from build123d import *

# Parameters (mm, degrees)
F1_DEPTH  = 2
F2_R      = 1.5
F3_DEPTH  = 5
F4_R      = 19
F5_DEPTH  = 27
F6_W      = 47
F6_H      = 27
F7_DEPTH  = 5
F8_W      = 47
F8_H      = 5
F9_DEPTH  = 120
F11_DEPTH = 10
F13_DEPTH = 25
F15_DEPTH = 25
F16_R     = 5


with BuildPart() as f1:
    # F0 (on Front) → F1 (new body)
    with BuildSketch(Plane.XZ):
        with BuildLine():
            Line((-23.5, -23.5), (0, -23.5))
            Line((0, -23.5), (23.5, -23.5))
            Line((23.5, -23.5), (23.5, 0))
            ThreePointArc((23.5, 0), (0, 23.5), (-23.5, 0))
            Line((-23.5, 0), (-23.5, -23.5))
        make_face()
    extrude(amount=F1_DEPTH)

    # F2 (on face) → F3 (cut)
    with BuildSketch(Plane.XZ.offset(2)):
        with Locations((15.5, 0)):
            Circle(F2_R)
        with Locations((7.75, 13.423394)):
            Circle(F2_R)
        with Locations((-7.75, 13.423394)):
            Circle(F2_R)
        with Locations((-15.5, 0)):
            Circle(F2_R)
        with Locations((-7.75, -13.423394)):
            Circle(F2_R)
        with Locations((7.75, -13.423394)):
            Circle(F2_R)
        with BuildLine():
            Line((6.5, -7), (6.5, 7))
            ThreePointArc((6.5, 7), (0, 13.5), (-6.5, 7))
            Line((-6.5, 7), (-6.5, -7))
            ThreePointArc((-6.5, -7), (0, -13.5), (6.5, -7))
        make_face()
    extrude(amount=-F3_DEPTH, mode=Mode.SUBTRACT)

    # F4 (on Front) → F5 (join)
    with BuildSketch(Plane.XZ):
        with BuildLine():
            ThreePointArc((23.5, 0), (0, 23.5), (-23.5, 0))
            Line((-23.5, 0), (-23.5, -23.5))
            Line((-23.5, -23.5), (23.5, -23.5))
            Line((23.5, -23.5), (23.5, 0))
        make_face()
        with Locations((0, -0.678439)):
            Circle(F4_R, mode=Mode.SUBTRACT)
    extrude(amount=F5_DEPTH)

    # F6 (on face) → F7 (join)
    with BuildSketch(Plane(origin=(0, 0, -23.5), x_dir=(1, 0, 0), z_dir=(0, 0, -1))):
        with Locations((0, 13.5)):
            Rectangle(F6_W, F6_H)
    extrude(amount=F7_DEPTH)

    # F8 (on face) → F9 (join)
    with BuildSketch(Plane(origin=(0, 0, -28.5), x_dir=(1, 0, 0), z_dir=(0, 0, -1))):
        with Locations((0, 2.5)):
            Rectangle(F8_W, F8_H)
    extrude(amount=F9_DEPTH)

    # F10 (on face) → F11 (join)
    with BuildSketch(Plane.XZ.offset(5)):
        Polygon((-2.6, -51), (-2.6, -43.5), (-2.6, -36), (-7.6, -36), (-7.6, -51), align=None)
        Polygon((2.6, -126), (2.6, -133.5), (2.6, -141), (7.6, -141), (7.6, -126), align=None)
        Polygon((2.6, -36), (2.6, -43.5), (2.6, -51), (7.6, -51), (7.6, -36), align=None)
        Polygon((-2.6, -141), (-2.6, -133.5), (-2.6, -126), (-7.6, -126), (-7.6, -141), align=None)
    extrude(amount=F11_DEPTH)

    # F12 (on face) → F13 (cut)
    with BuildSketch(Plane.YZ.offset(7.6)):
        with BuildLine():
            ThreePointArc((-9.16795, -42.251925), (-10, -42), (-10.83205, -42.251925))
            Line((-10.83205, -42.251925), (-10, -43.5))
            Line((-10, -43.5), (-9.16795, -42.251925))
        make_face()
        with BuildLine():
            Line((-10, -43.5), (-10.83205, -42.251925))
            ThreePointArc((-10.83205, -42.251925), (-11.5, -43.5), (-10.83205, -44.748075))
            Line((-10.83205, -44.748075), (-10, -43.5))
        make_face()
        with BuildLine():
            Line((-9.16795, -42.251925), (-10, -43.5))
            Line((-10, -43.5), (-9.16795, -44.748075))
            ThreePointArc((-9.16795, -44.748075), (-8.677488, -44.207787), (-8.5, -43.5))
            ThreePointArc((-8.5, -43.5), (-8.677488, -42.792213), (-9.16795, -42.251925))
        make_face()
        with BuildLine():
            Line((-9.16795, -44.748075), (-10, -43.5))
            Line((-10, -43.5), (-10.83205, -44.748075))
            ThreePointArc((-10.83205, -44.748075), (-10, -45), (-9.16795, -44.748075))
        make_face()
    extrude(amount=-F13_DEPTH, mode=Mode.SUBTRACT)

    # F14 (on face) → F15 (cut)
    with BuildSketch(Plane.YZ.offset(7.6)):
        with BuildLine():
            ThreePointArc((-9.16795, -132.251925), (-10, -132), (-10.83205, -132.251925))
            Line((-10.83205, -132.251925), (-10, -133.5))
            Line((-10, -133.5), (-9.16795, -132.251925))
        make_face()
        with BuildLine():
            Line((-10, -133.5), (-10.83205, -132.251925))
            ThreePointArc((-10.83205, -132.251925), (-11.5, -133.5), (-10.83205, -134.748075))
            Line((-10.83205, -134.748075), (-10, -133.5))
        make_face()
        with BuildLine():
            Line((-9.16795, -132.251925), (-10, -133.5))
            Line((-10, -133.5), (-9.16795, -134.748075))
            ThreePointArc((-9.16795, -134.748075), (-8.677488, -134.207787), (-8.5, -133.5))
            ThreePointArc((-8.5, -133.5), (-8.677488, -132.792213), (-9.16795, -132.251925))
        make_face()
        with BuildLine():
            Line((-9.16795, -134.748075), (-10, -133.5))
            Line((-10, -133.5), (-10.83205, -134.748075))
            ThreePointArc((-10.83205, -134.748075), (-10, -135), (-9.16795, -134.748075))
        make_face()
    extrude(amount=-F15_DEPTH, mode=Mode.SUBTRACT)

    # F16
    f16_edges = [f1.edges().sort_by_distance(p)[0] for p in [
        (5.1, -15, -141),
        (5.1, -15, -126),
        (-5.1, -15, -126),
        (-5.1, -15, -141),
        (5.1, -15, -51),
        (5.1, -15, -36),
        (-5.1, -15, -36),
        (-5.1, -15, -51),
    ]]
    fillet(f16_edges, radius=F16_R)


solid = f1.part
Work out the finished part from the listing and answer in its coordinate system (mm). A direction names the side the tool comes from. Give positions to 0.01 mm unless a question says otherwise; leave off trailing zeros. Order: outer loops, then holes, each group sorted by start corner. A loop starts at its lowest first (then second) coordinate and runs counter-clockwise, first axis right, second up. Notation, with made-up numbers: (-19, -6.5) -> (32, -6.5) arc R28 cw to (32, 23.5) -> close; hole circle Ø1 at (23.5, 29.5). An arc over 180 degrees is marked (long way). Answer as a JSON object with one key per item and string values. Group by question number.
1. Section A-A on x = 0 is taken. Determine the outline of the cut face in (y, z).
2. Section C-C on z = -53.5 is taken. Determine the outline of the cut face in (x, y), plus the area to 3 significant figures.
3. Section B-B on y = -25.5 is taken. Determine the outline of the cut face in (x, z), plus the area to 3 significant figures.
4. The mould has two halves that part along Z. Classify faces 6 (the flat face through (5, -7, -51)), 7 (the flat face through (-5, -15, -133)), 8 (the flat face through (-5, -7, -141)): released by +Z, released by -Z, zero draft, split by the parting line, or undercut.
5. Section D-D on x = 15.5 is taken. Determine the outline of the cut face in (y, z).
6. Flat-ended cylindrical pins translate along their axes: pin 1 Ø3 at (x, y) = (-6.5, -12.5) entering from +Z; pin 2 Ø1.5 at (x, y) = (-4, -8) entering from -Z; pin 3 Ø6 at (x, y) = (-13, -8.5) entering from +Z. Find the tip coordinate at first contact, or state that the pin passes through.
7. A tool of negligible diameter and unlimited length cuts with its end or side. For faces 1 (the flat face through (-7.6, -9.9, -131.7)), 2 (the cylindrical face through (-5, -13, -50)), 3 (the flat face through (5, -15, -43)), 4 (the flat face through (-2.6, -9.9, -45.3)), 5 (the cylindrical face through (0.1, -1, 13.5)), from which of +Z, -Z, +X, -X, +Y, -Y can it reach the whole face along a straight path? Write none if from no direction.
8. Consider line 1 along Z through (x, y) = (0, -17.5); line 2 along Z through (x, y) = (-7.75, -0.95); line 3 along Y through (x, z) = (13, -130). Determine where each line is inside the solid, lowest interval first. Write a range as [from, to].
Result sheet:
{
 "1": {"outline": "(-27, -28.5) -> (-5, -28.5) -> (-5, -148.5) -> (0, -148.5) -> (0, -13.5) -> (-2, -13.5) -> (-2, -19.68) -> (-27, -19.68) -> close; (-27, 18.32) -> (-2, 18.32) -> (-2, 13.5) -> (0, 13.5) -> (0, 23.5) -> (-27, 23.5) -> close"},
 "2": {"outline": "(-23.5, -5) -> (23.5, -5) -> (23.5, 0) -> (-23.5, 0) -> close", "area": "235 mm^2"},
 "3": {"outline": "(-23.5, -28.5) -> (23.5, -28.5) -> (23.5, 0) arc R23.5 ccw to (-23.5, 0) -> close; hole circle Ø38 at (0, -0.68)", "area": "1,070 mm^2"},
 "4": {"face 6": "undercut", "face 7": "zero draft", "face 8": "released by -Z"},
 "5": {"outline": "(-27, -28.5) -> (-5, -28.5) -> (-5, -148.5) -> (0, -148.5) -> (0, -1.5) -> (-2, -1.5) -> (-2, -11.67) -> (-27, -11.67) -> close; (-27, 10.31) -> (-2, 10.31) -> (-2, 1.5) -> (0, 1.5) -> (0, 17.66) -> (-27, 17.66) -> close"},
 "6": {"pin 1": "stops at z = 22.96", "pin 2": "stops at z = -141", "pin 3": "stops at z = 21.27"},
 "7": {"face 1": "-Z, -X, -Y", "face 2": "+X, -X, -Y", "face 3": "-Z, +X, -X, -Y", "face 4": "-Z, -Y", "face 5": "+Y, -Y"},
 "8": {"line 1": "z = [-28.5, -19.68], [18.32, 23.5]", "line 2": "z = [-148.5, -14.92], [-11.92, 11.92], [14.92, 22.19]", "line 3": "y = [-5, 0]"}
}
